```python
from build123d import *

# Parameters (mm, degrees)
SKETCH_W     = 130
SKETCH_H     = 68
PAD_DEPTH    = 1
SKETCH001_W  = 100
SKETCH001_H  = 1
PAD001_DEPTH = 28
SKETCH002_W  = 100
SKETCH002_H  = 1
PAD002_DEPTH = 28
PAD003_DEPTH = 28
SKETCH004_W  = 100
SKETCH004_H  = 2.7
PAD004_DEPTH = 25
SKETCH005_W  = 100
SKETCH005_H  = 1
PAD005_DEPTH = 3
SKETCH006_W  = 100
SKETCH006_H  = 1
PAD006_DEPTH = 3
PAD007_DEPTH = 3
PAD008_DEPTH = 15


with BuildPart() as part:
    # Sketch → Pad (new body)
    with BuildSketch(Plane.XY):
        with Locations((65, 34)):
            Rectangle(SKETCH_W, SKETCH_H)
    extrude(amount=-PAD_DEPTH)

    # Sketch001 → Pad001 (join)
    with BuildSketch(Plane.XY):
        with Locations((54, 56.8)):
            Rectangle(SKETCH001_W, SKETCH001_H)
    extrude(amount=PAD001_DEPTH)

    # Sketch002 → Pad002 (join)
    with BuildSketch(Plane.XY):
        with Locations((54, 60.5)):
            Rectangle(SKETCH002_W, SKETCH002_H)
    extrude(amount=PAD002_DEPTH)

    # Sketch003 → Pad003 (join)
    with BuildSketch(Plane.XY):
        Polygon((104, 61), (112, 65), (114, 65), (104, 60), align=None)
        Polygon((104, 57.3), (109, 55), (106.826087, 55), (104, 56.3), align=None)
    extrude(amount=PAD003_DEPTH)

    # Sketch004 → Pad004 (join)
    with BuildSketch(Plane.XY):
        with Locations((54, 58.65)):
            Rectangle(SKETCH004_W, SKETCH004_H)
    extrude(amount=PAD004_DEPTH)

    # Sketch005 → Pad005 (join)
    with BuildSketch(Plane.XY):
        with Locations((54, 7.5)):
            Rectangle(SKETCH005_W, SKETCH005_H)
    extrude(amount=PAD005_DEPTH)

    # Sketch006 → Pad006 (join)
    with BuildSketch(Plane.XY):
        with Locations((54, 11.2)):
            Rectangle(SKETCH006_W, SKETCH006_H)
    extrude(amount=PAD006_DEPTH)

    # Sketch007 → Pad007 (join)
    with BuildSketch(Plane.XY):
        Polygon((104, 10.7), (114, 19), (112.795181, 19), (104, 11.7), align=None)
        Polygon((104, 8), (114, 3.7), (111.674419, 3.7), (104, 7), align=None)
    extrude(amount=PAD007_DEPTH)

    # Sketch008 → Pad008 (join)
    with BuildSketch(Plane.XY):
        Polygon((60, 36.5), (63, 36.5), (63, 31.5), (60, 31.5), (60, 32.5), (62, 32.5), (62, 33.5), (60, 33.5), (60, 34.5), (62, 34.5), (62, 35.5), (60, 35.5), align=None)
    extrude(amount=PAD008_DEPTH)


solid = part.part
```
The listing builds one solid part. Answer for the finished solid, in the listing's coordinates (mm). A direction names the side the tool comes from. Give positions to 0.01 mm unless a question says otherwise; leave off trailing zeros. Loops run counter-clockwise (first coordinate to the right, second up) from the corner with the lowest first, then second, coordinate; pieces in that order, holes last. Notation, with made-up numbers: (24.5, 11.5) - (36.5, 11.5) arc R11 ccw to (36.5, 18.5) - close; hole circle Ø5 at (-15.75, 76). An arc over 180 degrees is marked (long way). Return JSON: item names as keys, results as strings. Group by question number.
1. Find section D-D (y = 17). Write down the section's boundary in (x, z), then the cut area to 3 significant figures.
2. Find section B-B (x = 65). Write down the section's boundary in (y, z).
3. Find section A-A (z = 12.75). Write down the section's boundary in (x, y), then the cut area to 3 significant figures.
4. Find section C-C (z = 22.25). Write down the section's boundary in (x, y), then the cut area to 3 significant figures.
5. Which of the six approach directions +Z, -Z, +X, -X, +Y, -Y give full straight-line access (tool end or side, diameter ignored) to faces 1 (the flat face through (104, 59, 12)), 2 (the flat face through (53, 10.7, 1)), 3 (the flat face through (113, 3.7, 1)), 4 (the flat face through (108.46, 15.4, 1.48))?
6. Given pin 1 Ø3.5 at (x, z) = (38, 26) entering from -Y; pin 2 Ø1 at (x, z) = (113.5, 2) entering from +Y; pin 3 Ø2 at (y, z) = (58.5, 14) entering from +X, each flat-ended and moving along its own axis, determine where each tip first touches the part or whether it passes through.
7. Determine the mould class of faces 5 (the flat face through (53, 11.7, 1)), 6 (the flat face through (61, 36.5, 7)), 7 (the flat face through (53, 7, 1)), 8 (the flat face through (4, 59, 14)) for opening direction Y: pulls with the +Y half, pulls with the -Y half, needs draft (parallel to the pull), parting line crosses it, or undercut.
8. Straight lines are drawn through the part: line 1 (Y direction, x = 50.5, z = 1.75); line 2 (Y direction, x = 76, z = 26.75); line 3 (Y direction, x = 96.5, z = 14.75). For each, find the intervals that lie inside material, in ascending order. Write a range as [from, to].
Verdict:
{
 "1": {"outline": "(0, -1) - (130, -1) - (130, 0) - (111.59, 0) - (111.59, 3) - (110.39, 3) - (110.39, 0) - (0, 0) - close", "area": "134 mm^2"},
 "2": {"outline": "(0, -1) - (68, -1) - (68, 0) - (61, 0) - (61, 28) - (60, 28) - (60, 25) - (57.3, 25) - (57.3, 28) - (56.3, 28) - (56.3, 0) - (11.7, 0) - (11.7, 3) - (10.7, 3) - (10.7, 0) - (8, 0) - (8, 3) - (7, 3) - (7, 0) - (0, 0) - close"},
 "3": {"outline": "(4, 56.3) - (104, 56.3) - (106.83, 55) - (109, 55) - (104, 57.3) - (104, 60) - (114, 65) - (112, 65) - (104, 61) - (4, 61) - close; (60, 31.5) - (63, 31.5) - (63, 36.5) - (60, 36.5) - (60, 35.5) - (62, 35.5) - (62, 34.5) - (60, 34.5) - (60, 33.5) - (62, 33.5) - (62, 32.5) - (60, 32.5) - close", "area": "494 mm^2"},
 "4": {"outline": "(4, 56.3) - (104, 56.3) - (106.83, 55) - (109, 55) - (104, 57.3) - (104, 60) - (114, 65) - (112, 65) - (104, 61) - (4, 61) - close", "area": "483 mm^2"},
 "5": {"face 1": "+Z, +X", "face 2": "+Z, +X, -X", "face 3": "+Z, +X, -X, -Y", "face 4": "+Z, -X"},
 "6": {"pin 1": "stops at y = 56.3", "pin 2": "stops at y = 65", "pin 3": "stops at x = 104"},
 "7": {"face 5": "undercut", "face 6": "undercut", "face 7": "pulls with the -Y half", "face 8": "needs draft"},
 "8": {"line 1": "y = [7, 8], [10.7, 11.7], [56.3, 61]", "line 2": "y = [56.3, 57.3], [60, 61]", "line 3": "y = [56.3, 61]"}
}
